Geometry check sheet. Reference: drawing and pictorial views, mm from the part's lowest x, y, z. Give positions to 0.01 mm unless a question says otherwise; leave off trailing zeros. Write each loop counter-clockwise with the first axis right and the second up, starting at its lowest first coordinate (ties: lowest second). Pieces come first, ordered by that corner, then holes. Notation, with made-up numbers: (47.25, 65.25) - (79.25, 65.25) arc R8 cw to (79.25, 71.25) - close; hole circle Ø9 at (75, 28.25). An arc over 180 degrees is marked (long way). Put each result on its own line as item: value.
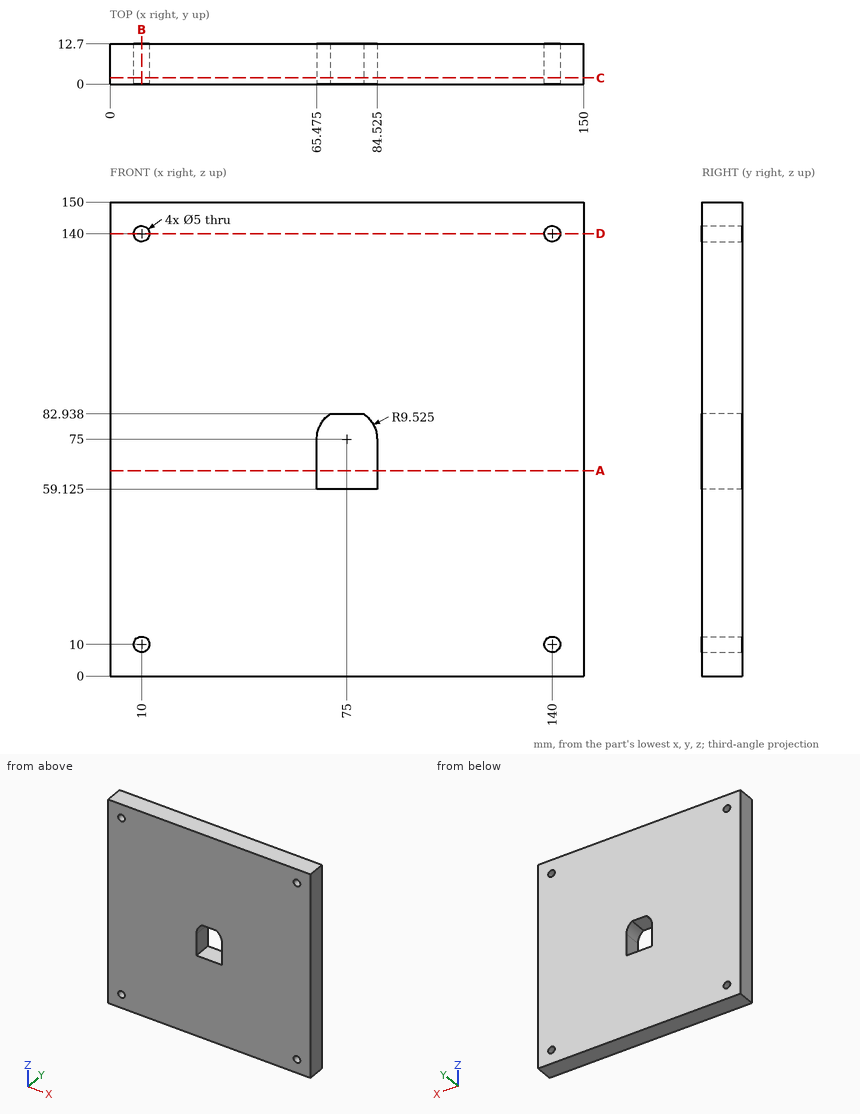
Q1. Section check D-D, the plane z = 140. Record the cut outline in (x, y), plus the area to 3 significant figures.
Answers follow:
outline: (0, 0) - (7.5, 0) - (7.5, 12.7) - (0, 12.7) - close; (12.5, 0) - (137.5, 0) - (137.5, 12.7) - (12.5, 12.7) - close; (142.5, 0) - (150, 0) - (150, 12.7) - (142.5, 12.7) - close
area: 1,780 mm2
Q2. Section check C-C, the plane y = 2. Give the number of separate pieces and of enclosed holes in the cut face, plus the area to 3 significant figures.
Answers follow:
separate pieces: 1
enclosed holes: 5
area: 22,000 mm2
Q3. Go/stop test with a flat-tipped pin: pin 1 Ø3 at (y, z) = (3, 54.5) entering from -X. Record where the tip stops, or that it passes through.
Answers follow:
pin 1: stops at x = 0
Q4. Scan lines: line 1 along X through (y, z) = (7.5, 140); line 2 along X through (y, z) = (2.25, 69.5) (1 decimal). Record each from-to range of solid material in increasing order.
Answers follow:
line 1: x = 0 to 7.5, 12.5 to 137.5, 142.5 to 150
line 2: x = 0 to 65.5, 84.5 to 150
Q5. Section check A-A, the plane z = 65. Record the cut outline in (x, y) (1 decimal), plus the area to 3 significant figures.
Answers follow:
outline: (0, 0) - (65.5, 0) - (65.5, 12.7) - (0, 12.7) - close; (84.5, 0) - (150, 0) - (150, 12.7) - (84.5, 12.7) - close
area: 1,660 mm2
Q6. Section check B-B, the plane x = 10. Record the cut outline in (y, z).
Answers follow:
outline: (0, 0) - (12.7, 0) - (12.7, 7.5) - (0, 7.5) - close; (0, 12.5) - (12.7, 12.5) - (12.7, 137.5) - (0, 137.5) - close; (0, 142.5) - (12.7, 142.5) - (12.7, 150) - (0, 150) - close
